Verification items for the finished model (mm, model axes). A direction names the side the tool comes from. Give positions to 0.01 mm unless a question says otherwise; leave off trailing zeros. Write each loop counter-clockwise with the first axis right and the second up, starting at its lowest first coordinate (ties: lowest second). Pieces come first, ordered by that corner, then holes. Notation, with made-up numbers: (-18.5, -21) -> (20.5, -21) arc R26 ccw to (20.5, 9) -> close; hole circle Ø9 at (35.25, -36). An arc over 180 degrees is marked (long way). Answer as CSV lines item,"result".
```python
from build123d import *

# Parameters (mm, degrees)
BOSS_EXTRUDE1_DEPTH = 10.16
SKETCH2_R           = 2.2857079
BOSS_EXTRUDE2_DEPTH = 5.588
SKETCH3_R           = 6.35
CUT_EXTRUDE1_DEPTH  = 10.16
SCALE1_SCALE        = 1.75


with BuildPart() as part:
    # Sketch1 → Boss-Extrude1 (new body)
    with BuildSketch(Plane.XY):
        with BuildLine():
            Line((-6.35, 25.4), (-6.35, 14.199031657))
            ThreePointArc((-6.35, 14.199031657), (-6.9032696, 11.606655013), (-8.466666667, 9.466021105))
            ThreePointArc((-8.466666667, 9.466021105), (-10.998522628, 6.35), (-12.431148083, 2.599337866))
            ThreePointArc((-12.431148083, 2.599337866), (-13.503292894, 0.175079336), (-15.471722124, -1.600254515))
            Line((-15.471722124, -1.600254515), (-25.172045256, -7.200738686))
            ThreePointArc((-25.172045256, -7.200738686), (-27.49630657, -15.875), (-18.822045256, -18.199261314))
            Line((-18.822045256, -18.199261314), (-9.121722124, -12.598777143))
            ThreePointArc((-9.121722124, -12.598777143), (-6.600023294, -11.781734349), (-3.964481416, -12.065358971))
            ThreePointArc((-3.964481416, -12.065358971), (0, -12.7), (3.964481416, -12.065358971))
            ThreePointArc((3.964481416, -12.065358971), (6.600023294, -11.781734349), (9.121722124, -12.598777143))
            Line((9.121722124, -12.598777143), (18.822045256, -18.199261314))
            ThreePointArc((18.822045256, -18.199261314), (27.49630657, -15.875), (25.172045256, -7.200738686))
            Line((25.172045256, -7.200738686), (15.471722124, -1.600254515))
            ThreePointArc((15.471722124, -1.600254515), (13.503292894, 0.175079336), (12.431148083, 2.599337866))
            ThreePointArc((12.431148083, 2.599337866), (10.998522628, 6.35), (8.466666667, 9.466021105))
            ThreePointArc((8.466666667, 9.466021105), (6.9032696, 11.606655013), (6.35, 14.199031657))
            Line((6.35, 14.199031657), (6.35, 25.4))
            ThreePointArc((6.35, 25.4), (0, 31.75), (-6.35, 25.4))
        make_face()
    extrude(amount=BOSS_EXTRUDE1_DEPTH)

    # Sketch2 → Boss-Extrude2 (add)
    with BuildSketch(Plane(origin=(0, 0, 0), x_dir=(-1, 0, 0), z_dir=(0, 0, -1))):
        with Locations((0, 25.4)):
            Circle(SKETCH2_R)
        with Locations((21.997045256, -12.7)):
            Circle(SKETCH2_R)
        with Locations((-21.997045256, -12.7)):
            Circle(SKETCH2_R)
    extrude(amount=BOSS_EXTRUDE2_DEPTH)

    # Sketch3 → Cut-Extrude1 (cut)
    with BuildSketch(Plane(origin=(0, 0, 0), x_dir=(-1, 0, 0), z_dir=(0, 0, -1))):
        Circle(SKETCH3_R)
    extrude(amount=-CUT_EXTRUDE1_DEPTH, mode=Mode.SUBTRACT)


with BuildPart() as part_1:
    # Scale1: scaled about (0, 0, 4.887896588)
    add(part.part.scale(SCALE1_SCALE).moved(Location((0, 0, -3.665922441))))


solid = part_1.part
```
1) Scan lines: line 1 along Z through (x, y) = (32, -6); line 2 along X through (y, z) = (6, 6.25); line 3 along Y through (x, z) = (-42.5, 7). Record each from-to range of solid material in increasing order.
Reported:
line 1,"-3.67 to 14.11"
line 2,"-21.4 to -9.35, 9.35 to 21.4"
line 3,"-32.59 to -11.71"
2) Section check C-C (y = 0). Record the boundary of the cut face in (x, z).
Reported:
outline,"(-23.86, -3.67) -> (-11.11, -3.67) -> (-11.11, 14.11) -> (-23.86, 14.11) -> close; (11.11, -3.67) -> (23.86, -3.67) -> (23.86, 14.11) -> (11.11, 14.11) -> close"
3) Section check D-D (z = -6). Record the boundary of the cut face in (x, y) (3 decimals), and give its area (3 significant figures).
Reported:
outline,"circle Ø8 at (-38.495, -22.225); circle Ø8 at (0, 44.45); circle Ø8 at (38.495, -22.225)"
area,"151 mm²"
4) Draft check along X on faces 5 (the cylindrical face through (11.48, -20.61, 5.1)), 6 (the flat face through (-11.112, 35, 5)), 7 (the flat face through (0, 45, -13.445)). Enter one of: +X half, -X half, draft (parallel to the pull), parting line (faces both ways), or undercut.
Reported:
face 5,"undercut"
face 6,"-X half"
face 7,"draft"
5) Tool access check on faces 1 (the flat face through (39, -22, -13.445)), 2 (the flat face through (24.33, -26.88, 5.1)), 3 (the flat face through (11.112, 35, 5)), 4 (the cylindrical face through (-34.5, -22, -8.5)). Record the directions out of +Z, -Z, +X, -X, +Y, -Y that give a thin tool (end or side, any length) a straight path to the whole face; none if there is none.
Reported:
face 1,"-Z, +X, -X, +Y, -Y"
face 2,"+Z, -Z, -Y"
face 3,"+Z, -Z, +X, +Y"
face 4,"-Z"
6) Depth check by flat-ended pin: pin 1 (3 mm diameter, centred on x = -4, z = 8.5, fed in from -Y); pin 2 (6 mm diameter, centred on x = -30, y = -2, fed in from -Z); pin 3 (6 mm diameter, centred on y = 23, z = 8, fed in from -X). Enter the tip coordinate at first touch or a pass-through.
Reported:
pin 1,"y = -22.08"
pin 2,"z = -3.67"
pin 3,"x = -12.23"
7) Section check A-A (x = 0). Record the boundary of the cut face in (y, z) (1 decimal), and give its area (3 significant figures).
Reported:
outline,"(-22.2, -3.7) -> (-11.1, -3.7) -> (-11.1, 14.1) -> (-22.2, 14.1) -> close; (11.1, -3.7) -> (40.5, -3.7) -> (40.5, -13.4) -> (48.4, -13.4) -> (48.4, -3.7) -> (55.6, -3.7) -> (55.6, 14.1) -> (11.1, 14.1) -> close"
area,"1,070 mm²"
